from build123d import *

# Parameters (mm, degrees)
ESQUISSE1_W        = 200
ESQUISSE1_H        = 180
ESQUISSE1_R        = 10
BOSS_EXTRU_1_DEPTH = 10
ESQUISSE3_R        = 10
BOSS_EXTRU_2_DEPTH = 50
ESQUISSE4_W        = 20
ESQUISSE4_H        = 10
BOSS_EXTRU_3_DEPTH = 10
CONG_1_R           = 1


with BuildPart() as part:
    # Esquisse1 → Boss.-Extru.1 (new body)
    with BuildSketch(Plane.XY):
        Rectangle(ESQUISSE1_W, ESQUISSE1_H)
        with Locations((-30, 0)):
            Circle(ESQUISSE1_R, mode=Mode.SUBTRACT)
    extrude(amount=BOSS_EXTRU_1_DEPTH)

    # Esquisse3 → Boss.-Extru.2 (add)
    with BuildSketch(Plane(origin=(0, 0, 0), x_dir=(-1, 0, 0), z_dir=(0, 0, -1))):
        with Locations((30, 0)):
            Circle(ESQUISSE3_R)
    extrude(amount=-BOSS_EXTRU_2_DEPTH)

    # Esquisse4 → Boss.-Extru.3 (add)
    with BuildSketch(Plane.XY.offset(10)):
        with Locations((-80, -20)):
            Rectangle(ESQUISSE4_W, ESQUISSE4_H)
        Polygon((-12.32233047, -38.890872965), (1.819805153, -53.033008589), (-5.251262658, -60.104076401), (-19.393398282, -45.961940777), align=None)
    extrude(amount=BOSS_EXTRU_3_DEPTH)

    # Congé1
    cong_1_edges = [part.edges().sort_by_distance(p)[0] for p in [
        (-70, -15, 15),
        (-12.32233047, -38.890872965, 15),
    ]]
    fillet(cong_1_edges, radius=CONG_1_R)


solid = part.part
The model under review builds one solid part; all positions refer to its coordinate system, in mm. A direction names the side the tool comes from. Coordinates: 2 decimals unless noted, no trailing zeros. Write each loop counter-clockwise with the first axis right and the second up, starting at its lowest first coordinate (ties: lowest second). Pieces come first, ordered by that corner, then holes. Notation, with made-up numbers: (-22.75, 57.25) -> (26.25, 57.25) arc R30 ccw to (26.25, 83.25) -> close; hole circle Ø3 at (9.5, 22). An arc over 180 degrees is marked (long way). Answer in a Markdown table with one row per item.
1. Clearance check with flat-ended pins moving along their axes: pin 1 Ø2 at (x, z) = (-15, 19) entering from -Y; pin 2 Ø1 at (x, y) = (41.5, 28) entering from +Z; pin 3 Ø10.5 at (x, y) = (-10, -53.5) entering from +Z. State where each tip first meets the part, or that it passes through.
Answers below:
| item | result |
|---|---|
| pin 1 | stops at y = -51.36 |
| pin 2 | stops at z = 10 |
| pin 3 | stops at z = 20 |
2. We need section B-B, the plane x = -86.5. State the section outline as (y, z) points.
Answers below:
| item | result |
|---|---|
| outline | (-90, 0) -> (90, 0) -> (90, 10) -> (-15, 10) -> (-15, 20) -> (-25, 20) -> (-25, 10) -> (-90, 10) -> close |
3. Wall thickness on probe 1 along Z at (x, y) = (60, 33); probe 2 along X at (y, z) = (-51.5, 16.5); probe 3 along X at (y, z) = (-6.5, 44): over which ranges is each line inside the solid? List them lowest first. Write a range as [from, to].
Answers below:
| item | result |
|---|---|
| probe 1 | z = [0, 10] |
| probe 2 | x = [-13.86, 0.29] |
| probe 3 | x = [-37.6, -22.4] |
4. We need section D-D, the plane z = 33.5. State the section outline as (x, y) points.
Answers below:
| item | result |
|---|---|
| outline | circle Ø20 at (-30, 0) |
5. We need section C-C, the plane y = 0. State the section outline as (x, z) points, and give its area (3 significant figures).
Answers below:
| item | result |
|---|---|
| outline | (-100, 0) -> (100, 0) -> (100, 10) -> (-20, 10) -> (-20, 50) -> (-40, 50) -> (-40, 10) -> (-100, 10) -> close |
| area | 2,800 mm^2 |
6. For faces 1 (the flat face through (-12.223, -53.132, 14.93)), 2 (the flat face through (-4.992, -46.221, 14.93)), 3 (the flat face through (-1.67, -56.52, 14.93)), list the 3-axis set-ups (+Z, -Z, +X, -X, +Y, -Y) from which the entire face can be reached by the end or side of a thin tool; tool diameter is ignored.
Answers below:
| item | result |
|---|---|
| face 1 | +Z, -X, -Y |
| face 2 | +Z, +X, +Y |
| face 3 | +Z, +X, -Y |
7. We need section A-A, the plane z = 17.5. State the section outline as (x, y) points.
Answers below:
| item | result |
|---|---|
| outline | (-90, -25) -> (-70, -25) -> (-70, -16) arc R1 ccw to (-71, -15) -> (-90, -15) -> close; circle Ø20 at (-30, 0); (-19.39, -45.96) -> (-5.25, -60.1) -> (1.82, -53.03) -> (-11.62, -39.6) arc R1 ccw to (-13.03, -39.6) -> close |
